Part model, mm, in its own coordinate system. A direction names the side the tool comes from. Give positions to 0.01 mm unless a question says otherwise; leave off trailing zeros. Write each loop counter-clockwise with the first axis right and the second up, starting at its lowest first coordinate (ties: lowest second). Pieces come first, ordered by that corner, then holes.
```python
from build123d import *

# Parameters (mm, degrees)
F1_DEPTH = 80
F2_W     = 178.746274
F2_H     = 66.143535
F3_DEPTH = 25
F4_R     = 50
F5_DEPTH = 25


with BuildPart() as f1:
    # F0 (on Front) → F1 (new body, symmetric)
    with BuildSketch(Plane.XZ):
        Polygon((-151.933498, 133.443999), (-151.933498, 15.624951), (-151.933498, -106.556001), (168.066502, -106.556001), (168.066502, -86.556001), (-131.933498, -86.556001), (-131.933498, 133.443999), align=None)
    extrude(amount=F1_DEPTH, both=True)

    # F2 (on face) → F3 (cut)
    with BuildSketch(Plane.XY.offset(-86.556001)):
        with Locations((78.693365, -1.327616)):
            Rectangle(F2_W, F2_H)
    extrude(amount=-F3_DEPTH, mode=Mode.SUBTRACT)

    # F4 (on face) → F5 (join)
    with BuildSketch(Plane(origin=(-151.933498, 0, 0), x_dir=(0, -1, 0), z_dir=(-1, 0, 0))):
        Circle(F4_R)
    extrude(amount=F5_DEPTH)


solid = f1.part
```
1) Saw through at D-D, the plane x = -50. Write the cut outline in (y, z).
Answers follow:
outline: (-80, -106.56) - (80, -106.56) - (80, -86.56) - (-80, -86.56) - close
2) Saw through at C-C, the plane y = 10.5. Write the cut outline in (x, z), then the cut area to 3 significant figures.
Answers follow:
outline: (-176.93, -48.89) - (-151.93, -48.89) - (-151.93, -106.56) - (-10.68, -106.56) - (-10.68, -86.56) - (-131.93, -86.56) - (-131.93, 133.44) - (-151.93, 133.44) - (-151.93, 48.89) - (-176.93, 48.89) - close
area: 9,670 mm2
3) Two-plate mould, pull along Y, no slides. Class faces 6 (the face through (168.067, -58, -97)), 7 (the face through (-10.68, -2, -96)), 8 (the face through (-64, 80, -93)), 9 (the face through (77, 31.744, -96)): +Y half, -Y half, draft (parallel to the pull), parting line (faces both ways), or undercut.
Answers follow:
face 6: draft
face 7: undercut
face 8: +Y half
face 9: undercut
4) Saw through at A-A, the plane x = 18.5. Write the cut outline in (y, z), then the cut area to 3 significant figures.
Answers follow:
outline: (-80, -106.56) - (-34.4, -106.56) - (-34.4, -86.56) - (-80, -86.56) - close; (31.74, -106.56) - (80, -106.56) - (80, -86.56) - (31.74, -86.56) - close
area: 1,880 mm2
5) Wall check: L1, parallel to X at y = -46, z = -55.5; L2, parallel to Z at x = -77.5, y = -0.5. Give the ranges that are in metal, low to high.
Answers follow:
L1: x = -151.93 to -131.93
L2: z = -106.56 to -86.56
6) Pin check, flat tips, straight feed: pin 1 Ø2 at (x, y) = (67.5, 50.5) entering from +Z; pin 2 Ø6 at (y, z) = (9.5, -93) entering from +X; pin 3 Ø3 at (y, z) = (-21.5, -80.5) entering from -X. Stop position of each tip, or through.
Answers follow:
pin 1: stops at z = -86.56
pin 2: stops at x = -10.68
pin 3: stops at x = -151.93
7) Saw through at B-B, the plane z = 0. Write the cut outline in (x, y), then the cut area to 3 significant figures.
Answers follow:
outline: (-176.93, -50) - (-151.93, -50) - (-151.93, -80) - (-131.93, -80) - (-131.93, 80) - (-151.93, 80) - (-151.93, 50) - (-176.93, 50) - close
area: 5,700 mm2
8) 3-axis set-ups, long thin cutter, end or side, ignore diameter. For faces 1 (the face through (-176.933, 1, 1)), 2 (the face through (-164.26, -47.69, 15.02)), 3 (the face through (168.067, 56, -97)), 4 (the face through (-13, -1, -86.556)), 5 (the face through (77, -34.399, -96)): which of +Z, -Z, +X, -X, +Y, -Y reach the whole face in a straight line?
Answers follow:
face 1: +Z, -Z, -X, +Y, -Y
face 2: -X
face 3: +Z, -Z, +X, +Y, -Y
face 4: +Z, +X, +Y, -Y
face 5: +Z, -Z, +X
